Geometry: see drawing. Coordinates: mm, zero at the bounding-box minimum. Round coordinates to 2 decimals unless told otherwise and drop trailing zeros. Loops run counter-clockwise (first coordinate to the right, second up) from the corner with the lowest first, then second, coordinate; pieces in that order, holes last. Notation, with made-up numbers: (79, 79) -> (102, 79) arc R14 cw to (102, 102) -> close; hole circle Ø7 at (3, 21). An arc over 180 degrees is marked (long way). Answer in a Markdown table with one row per item.
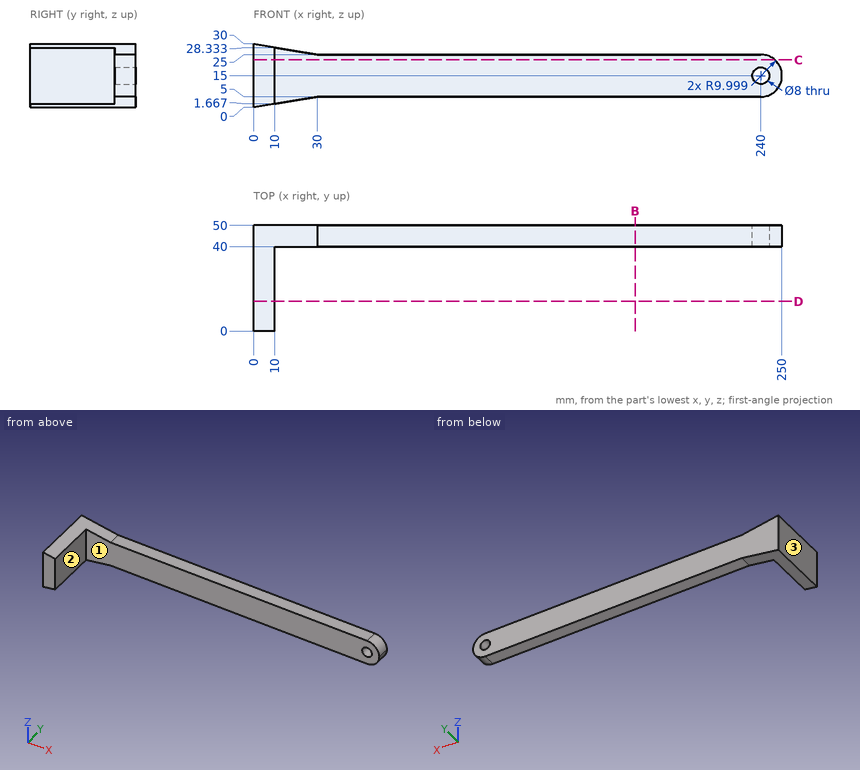
Item 1: Section query D-D, the plane y = 14. Output: boundary loops of the cut face in (x, z), and give its area (3 significant figures).
Ans:
| item | result |
|---|---|
| outline | (0, 0) -> (10, 1.67) -> (10, 28.33) -> (0, 30) -> close |
| area | 283 mm2 |
Item 2: Mould query, pull axis X, two halves, no side actions, for the marked faces 1, 2 and 3. Classes: released by +X, released by -X, zero draft, split by the parting line, or undercut.
Ans:
| item | result |
|---|---|
| face 1 | zero draft |
| face 2 | released by +X |
| face 3 | released by -X |
Item 3: Section query C-C, the plane z = 22.5. Output: boundary loops of the cut face in (x, y) (1 decimal).
Ans:
| item | result |
|---|---|
| outline | (0, 0) -> (10, 0) -> (10, 40) -> (246.6, 40) -> (246.6, 50) -> (0, 50) -> close |
Item 4: Section query B-B, the plane x = 180.5. Output: boundary loops of the cut face in (y, z), and give its area (3 significant figures).
Ans:
| item | result |
|---|---|
| outline | (40, 5) -> (50, 5) -> (50, 25) -> (40, 25) -> close |
| area | 200 mm2 |
Item 5: Ray query, L1, parallel to Z at x = 240, y = 44.75; L2, parallel to X at y = 45.25, z = 15; L3, parallel to X at y = 36, z = 14.25. Return the intervals inside material, ascending.
Ans:
| item | result |
|---|---|
| L1 | 5 to 11, 19 to 25 |
| L2 | 0 to 236, 244 to 250 |
| L3 | 0 to 10 |
Item 6: First-contact query: P1, Ø10, axis at x = 80, z = 16.5, coming from the -Y side; P2, Ø11, axis at x = 143.5, y = 46, coming from the -Z side; P3, Ø1.5, axis at y = 5, z = 4.5, coming from the +X side. Flat tips, straight axial feed; report the tip coordinate or a pass-through.
Ans:
| item | result |
|---|---|
| P1 | y = 40 |
| P2 | z = 5 |
| P3 | x = 10 |
